Could you check a few things on this model? Use its own coordinates, in mm. A direction names the side the tool comes from. Give positions to 0.01 mm unless a question says otherwise; leave off trailing zeros. Order: outer loops, then holes, each group sorted by start corner. A loop starts at its lowest first (then second) coordinate and runs counter-clockwise, first axis right, second up. Notation, with made-up numbers: (64, 60.5) -> (100, 60.5) arc R23 cw to (100, 91.5) -> close; hole circle Ø10 at (80, 36). An arc over 180 degrees is marked (long way). Write each question's results on one line, items separated by ' | '.
```python
from build123d import *

# Parameters (mm, degrees)
F1_DEPTH = 100
F3_D     = 11


with BuildPart() as f1:
    # F0 (on Top) → F1 (new body)
    with BuildSketch(Plane.XY):
        with BuildLine():
            Line((45, -298.3239697419), (45, -151.9868415357))
            ThreePointArc((45, -151.9868415357), (45.9495370635, -149.0553316858), (48.4375, -147.2372527377))
            ThreePointArc((48.4375, -147.2372527377), (155, 0), (48.4375, 147.2372527377))
            ThreePointArc((48.4375, 147.2372527377), (45.9495370635, 149.0553316858), (45, 151.9868415357))
            Line((45, 151.9868415357), (45, 298.3239697419))
            Line((45, 298.3239697419), (40, 298.3239697419))
            Line((40, 298.3239697419), (40, 144.568322948))
            ThreePointArc((40, 144.568322948), (149.8888164954, 1.8456395549), (43.5443348323, -143.5371914998))
            ThreePointArc((43.5443348323, -143.5371914998), (40.9826422963, -145.343888573), (40, -148.3206043943))
            Line((40, -148.3206043943), (40, -298.3239697419))
            Line((40, -298.3239697419), (45, -298.3239697419))
        make_face()
    extrude(amount=F1_DEPTH)

    # F3 (through all)
    with Locations(Plane.XZ.offset(298.3239697419)):
        with Locations((100, 89), (100, 11)):
            Hole(F3_D / 2)


solid = f1.part
```
Q1. Suppose I cut it at A-A on x = 62. Please give me the cut outline in (y, z).
Here are the results:
outline: (-142.06, 0) -> (-136.57, 0) -> (-136.57, 100) -> (-142.06, 100) -> close; (136.57, 0) -> (142.06, 0) -> (142.06, 100) -> (136.57, 100) -> close
Q2. Suppose I cut it at B-B on z = 89. Please give me the cut outline in (x, y), and give its area (3 significant figures).
Here are the results:
outline: (40, -298.32) -> (45, -298.32) -> (45, -151.99) arc R5 cw to (48.44, -147.24) arc R155 ccw to (94.5, -122.86) -> (94.5, -116.43) arc R150.04 cw to (43.54, -143.54) arc R5 ccw to (40, -148.32) -> close; (40, 144.57) arc R150.04 cw to (94.5, 116.43) -> (94.5, 122.86) arc R155 ccw to (48.44, 147.24) arc R5 cw to (45, 151.99) -> (45, 298.32) -> (40, 298.32) -> close; (105.5, -113.56) arc R155 ccw to (105.5, 113.56) -> (105.5, 106.55) arc R150.04 cw to (105.5, -106.55) -> close | area: 3,360 mm²
Q3. Thinking about a two-plate mould opening in Z: for faces 1 (the flat face through (153, 1, 100)), 2 (the cylindrical face through (97.043, 114.817, 93.638)), 3 (the flat face through (40, 223, 49)), which applies, +Z half, -Z half, draft (parallel to the pull), parting line (faces both ways), or undercut?
Here are the results:
face 1: +Z half | face 2: undercut | face 3: draft
Q4. I'm going to push flat-ended pins straight in: pin 1 Ø4 at (y, z) = (-206, 74) entering from +X; pin 2 Ø12 at (x, z) = (120.5, 48) entering from +Y; pin 3 Ø12.5 at (x, z) = (100, 89) entering from -Y; pin 4 Ø10 at (x, z) = (100, 11) entering from +Y. Where does each tip first touch, or does it pass through?
Here are the results:
pin 1: stops at x = 45 | pin 2: stops at y = 104.47 | pin 3: stops at y = -123.43 | pin 4: passes through
Q5. I need wall thicknesses on line 1 along Z through (x, y) = (100, -117); line 2 along Y through (x, z) = (72.5, 14.5); line 3 along Y through (x, z) = (132, 42.5). Which ranges of each line are inside material? Lowest first, please.
Here are the results:
line 1: z = 0 to 5.5, 16.5 to 83.5, 94.5 to 100 | line 2: y = -137 to -131.28, 131.28 to 137 | line 3: y = -81.25 to -71.07, 71.07 to 81.25
Q6. Suppose I cut it at D-D on z = 65.5. Please give me the cut outline in (x, y), and give its area (3 significant figures).
Here are the results:
outline: (40, -298.32) -> (45, -298.32) -> (45, -151.99) arc R5 cw to (48.44, -147.24) arc R155 ccw to (48.44, 147.24) arc R5 cw to (45, 151.99) -> (45, 298.32) -> (40, 298.32) -> (40, 144.57) arc R150.04 cw to (43.54, -143.54) arc R5 ccw to (40, -148.32) -> close | area: 3,510 mm²
Q7. Suppose I cut it at C-C on x = 100. Please give me the cut outline in (y, z), and give its area (3 significant figures).
Here are the results:
outline: (-118.43, 0) -> (-111.73, 0) -> (-111.73, 5.5) -> (-118.43, 5.5) -> close; (-118.43, 16.5) -> (-111.73, 16.5) -> (-111.73, 83.5) -> (-118.43, 83.5) -> close; (-118.43, 94.5) -> (-111.73, 94.5) -> (-111.73, 100) -> (-118.43, 100) -> close; (111.73, 0) -> (118.43, 0) -> (118.43, 5.5) -> (111.73, 5.5) -> close; (111.73, 16.5) -> (118.43, 16.5) -> (118.43, 83.5) -> (111.73, 83.5) -> close; (111.73, 94.5) -> (118.43, 94.5) -> (118.43, 100) -> (111.73, 100) -> close | area: 1,040 mm²
Q8. For faces 4 (the flat face through (45, 224, 49)), 5 (the cylindrical face through (149.83, 4.55, 49.3)), 6 (the flat face through (45, -226, 49)), which set-ups out of +Z, -Z, +X, -X, +Y, -Y let a thin tool reach every point of the face, with its end or its side?
Here are the results:
face 4: +Z, -Z, +X, +Y | face 5: +Z, -Z, -X | face 6: +Z, -Z, +X, -Y
